Could you check a few things on this model? Use its own coordinates, in mm. Give positions to 0.01 mm unless a question says otherwise; leave off trailing zeros. Write each loop counter-clockwise with the first axis right and the second up, starting at its lowest first coordinate (ties: lowest second). Pieces come first, ordered by that corner, then holes. Notation, with made-up numbers: (-4.75, 58.25) - (41.25, 58.25) arc R23 ccw to (41.25, 87.25) - close; hole circle Ø9 at (-10, 67.5). An arc over 180 degrees is marked (long way). Use one line per item in the form item = value.
```python
from build123d import *

# Parameters (mm, degrees)
SKETCH_1_R               = 29.5
EXTRUDE_1_DEPTH          = 3
HOLE_WIZARD_M3_4_D       = 2.5
HOLE_WIZARD_M3_1_D       = 2.5
SKETCH_9_R               = 2.75
CUT_EXTRUDE_1_DEPTH      = 1
CUT_EXTRUDE_1_DEPTH_BACK = 1


with BuildPart() as part:
    # 草图1 → 凸台-拉伸1 (new body)
    with BuildSketch(Plane(origin=(0, 0, 0), x_dir=(1, 0, 0), z_dir=(0, 1, 0))):
        Circle(SKETCH_1_R)
    extrude(amount=EXTRUDE_1_DEPTH)

    # M3 螺纹孔4 (through all)
    with Locations(Plane(origin=(0, 3, 0), x_dir=(1, 0, 0), z_dir=(0, 1, 0))):
        with Locations((6.180339887, 19.021130326), (20, 0), (6.180339887, -19.021130326), (-16.180339887, -11.755705046), (-16.180339887, 11.755705046)):
            Hole(HOLE_WIZARD_M3_4_D / 2)

    # M3 螺纹孔1 (through all)
    with Locations(Plane(origin=(0, 3, 0), x_dir=(1, 0, 0), z_dir=(0, 1, 0))):
        with Locations((20.225424859, -14.694631307), (-25, 0), (-7.071067812, 0), (-7.725424859, 23.776412907), (20.225424859, 14.694631307), (-7.725424859, -23.776412907), (0, 0), (0, 7.071067812), (7.071067812, 0), (0, -7.071067812)):
            Hole(HOLE_WIZARD_M3_1_D / 2)

    # 草图9 → 切除-拉伸1 (cut, two sides)
    with BuildSketch(Plane(origin=(0, 3, 0), x_dir=(1, 0, 0), z_dir=(0, 1, 0))) as cut_extrude_1_sk:
        with Locations((20, 0)):
            Circle(SKETCH_9_R)
        with Locations((6.180339887, -19.021130326)):
            Circle(SKETCH_9_R)
        with Locations((-16.180339887, -11.755705046)):
            Circle(SKETCH_9_R)
        with Locations((-16.180339887, 11.755705046)):
            Circle(SKETCH_9_R)
        with Locations((6.180339887, 19.021130326)):
            Circle(SKETCH_9_R)
    extrude(amount=CUT_EXTRUDE_1_DEPTH, mode=Mode.SUBTRACT)
    extrude(cut_extrude_1_sk.sketch, amount=-CUT_EXTRUDE_1_DEPTH_BACK, mode=Mode.SUBTRACT)


solid = part.part
```
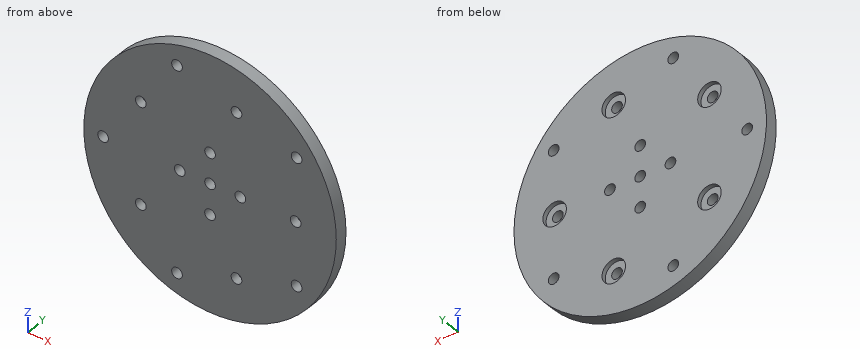
1. For pin 1 (2 mm diameter, centred on x = 0, z = 0, fed in from +Y); pin 2 (3 mm diameter, centred on x = 6.18, z = 19.02, fed in from +Y), each with a flat end and sliding along its axis, tell me the tip position at first contact or that it passes through.
Response values:
pin_1 = through
pin_2 = 2
2. If I drill on line 1 (X direction, y = 0.75, z = 1); line 2 (Z direction, x = -17, y = 2.65); line 3 (X direction, y = 0.65, z = 15.5), over which ranges is the centre line in solid material (lowest first)? Write a range as from..to.
Response values:
line_1 = -29.48..-25.75, -24.25..-7.82, -6.32..-0.75, 0.75..6.32, 7.82..19.25, 20.75..29.48
line_2 = -24.11..-14.38, -9.13..9.13, 14.38..24.11
line_3 = -25.1..19.27, 21.18..25.1
3. Imagine slicing it at C-C, the plane x = -25. List the corners of the cut face in (y, z) for me, and give its area (3 significant figures).
Response values:
outline = (0, -15.66) - (3, -15.66) - (3, -1.25) - (0, -1.25) - close; (0, 1.25) - (3, 1.25) - (3, 15.66) - (0, 15.66) - close
area = 86.5 mm²
4. Imagine slicing it at B-B, the plane x = 0. List the corners of the cut face in (y, z) for me, and give its area (4 significant figures).
Response values:
outline = (0, -29.5) - (3, -29.5) - (3, -8.32) - (0, -8.32) - close; (0, -5.82) - (3, -5.82) - (3, -1.25) - (0, -1.25) - close; (0, 1.25) - (3, 1.25) - (3, 5.82) - (0, 5.82) - close; (0, 8.32) - (3, 8.32) - (3, 29.5) - (0, 29.5) - close
area = 154.5 mm²
5. Imagine slicing it at A-A, the plane z = 0. List the corners of the cut face in (x, y) for me, and give its area (4 significant figures).
Response values:
outline = (-29.5, 0) - (-26.25, 0) - (-26.25, 3) - (-29.5, 3) - close; (-23.75, 0) - (-8.32, 0) - (-8.32, 3) - (-23.75, 3) - close; (-5.82, 0) - (-1.25, 0) - (-1.25, 3) - (-5.82, 3) - close; (1.25, 0) - (5.82, 0) - (5.82, 3) - (1.25, 3) - close; (8.32, 0) - (18.75, 0) - (18.75, 2) - (17.25, 2) - (17.25, 3) - (8.32, 3) - close; (21.25, 0) - (29.5, 0) - (29.5, 3) - (22.75, 3) - (22.75, 2) - (21.25, 2) - close
area = 136.5 mm²
6. Imagine slicing it at D-D, the plane y = 2.55. State how many separate pieces and enclosed holes the cut face has, and give its area (3 significant figures).
Response values:
separate_pieces = 1
enclosed_holes = 15
area = 2,570 mm²
